Verification items for the finished model (mm, model axes). Give positions to 0.01 mm unless a question says otherwise; leave off trailing zeros. Loops run counter-clockwise (first coordinate to the right, second up) from the corner with the lowest first, then second, coordinate; pieces in that order, holes last. Notation, with made-up numbers: (73, 36.25) - (122, 36.25) arc R28 cw to (122, 69.25) - close; hole circle Ø9 at (-11.75, 73). An arc over 180 degrees is marked (long way). Answer in a Markdown table with one row per item.
```python
from build123d import *

# Parameters (mm, degrees)
SKETCH1_R           = 11.43
BOSS_EXTRUDE1_DEPTH = 2
SKETCH2_W           = 17.3
SKETCH2_H           = 1
SKETCH2_W_2         = 1
SKETCH2_H_2         = 17.3
CUT_EXTRUDE7_DEPTH  = 2
SKETCH3_R           = 9.65
BOSS_EXTRUDE2_DEPTH = 10
SKETCH4_R           = 8.65
CUT_EXTRUDE8_DEPTH  = 10


with BuildPart() as part:
    # Sketch1 → Boss-Extrude1 (new body)
    with BuildSketch(Plane(origin=(0, 0, 0), x_dir=(1, 0, 0), z_dir=(0, 1, 0))):
        with Locations(Location((0, 0, 0), (0, 0, 270))):
            Circle(SKETCH1_R)
    extrude(amount=BOSS_EXTRUDE1_DEPTH)

    # Sketch2 → Cut-Extrude7 (cut)
    with BuildSketch(Plane(origin=(0, 2, 0), x_dir=(1, 0, 0), z_dir=(0, 1, 0))):
        Polygon((-6.470027048, 5.762920267), (5.762920267, -6.470027048), (6.470027048, -5.762920267), (-5.762920267, 6.470027048), align=None)
        Rectangle(SKETCH2_W, SKETCH2_H)
        Rectangle(SKETCH2_W_2, SKETCH2_H_2)
        Polygon((5.762920267, 6.470027048), (-6.470027048, -5.762920267), (-5.762920267, -6.470027048), (6.470027048, 5.762920267), align=None)
    extrude(amount=-CUT_EXTRUDE7_DEPTH, mode=Mode.SUBTRACT)

    # Sketch3 → Boss-Extrude2 (add)
    with BuildSketch(Plane(origin=(0, 2, 0), x_dir=(1, 0, 0), z_dir=(0, 1, 0))):
        with Locations(Location((0, 0, 0), (0, 0, 270))):
            Circle(SKETCH3_R)
    extrude(amount=BOSS_EXTRUDE2_DEPTH)

    # Sketch4 → Cut-Extrude8 (cut)
    with BuildSketch(Plane(origin=(0, 12, 0), x_dir=(1, 0, 0), z_dir=(0, 1, 0))):
        with Locations(Location((0, 0, 0), (0, 0, 270))):
            Circle(SKETCH4_R)
    extrude(amount=-CUT_EXTRUDE8_DEPTH, mode=Mode.SUBTRACT)


solid = part.part
```
Q1. Draft check along Z on faces 1 (the face through (8, 12, -4)), 2 (the face through (3, 2, 6)), 3 (the face through (-3.168, 1.014, 3.875)). Enter one of: +Z half, -Z half, draft (parallel to the pull), parting line (faces both ways), or undercut.
Completed:
| item | result |
|---|---|
| face 1 | draft |
| face 2 | undercut |
| face 3 | undercut |
Q2. Sectioned sample at B-B (z = 5). Record the cut outline in (x, y), and give its area (3 significant figures).
Completed:
| item | result |
|---|---|
| outline | (-10.28, 0) - (-5.71, 0) - (-5.71, 2) - (-7.06, 2) - (-7.06, 12) - (-8.25, 12) - (-8.25, 2) - (-10.28, 2) - close; (-4.29, 0) - (-0.5, 0) - (-0.5, 2) - (-4.29, 2) - close; (0.5, 0) - (4.29, 0) - (4.29, 2) - (0.5, 2) - close; (5.71, 0) - (10.28, 0) - (10.28, 2) - (8.25, 2) - (8.25, 12) - (7.06, 12) - (7.06, 2) - (5.71, 2) - close |
| area | 57.4 mm^2 |
Q3. Sectioned sample at D-D (x = -8). Record the cut outline in (y, z).
Completed:
| item | result |
|---|---|
| outline | (0, -8.16) - (2, -8.16) - (2, -5.4) - (12, -5.4) - (12, -3.29) - (2, -3.29) - (2, -0.5) - (0, -0.5) - close; (0, 0.5) - (2, 0.5) - (2, 3.29) - (12, 3.29) - (12, 5.4) - (2, 5.4) - (2, 8.16) - (0, 8.16) - close |
Q4. Go/stop test with flat-tipped pins: P1, Ø2.5, axis at x = 3.5, z = 4, coming from the +Y side; P2, Ø1, axis at x = 4.5, y = 1.5, coming from the +Z side; P3, Ø1.5, axis at y = 10.5, z = 3, coming from the -X side. Record where each tip stops, or that it passes through.
Completed:
| item | result |
|---|---|
| P1 | y = 2 |
| P2 | z = 10.71 |
| P3 | x = -9.38 |
Q5. Thickness scan on line 1 (X direction, y = 6.5, z = 0); line 2 (Y direction, x = -8.25, z = -7). Record the ranges inside material, lowest first.
Completed:
| item | result |
|---|---|
| line 1 | -9.65 to -8.65, 8.65 to 9.65 |
| line 2 | 0 to 2 |
Q6. Sectioned sample at A-A (x = -4.25). Record the cut outline in (y, z), and give its area (3 significant figures).
Completed:
| item | result |
|---|---|
| outline | (0, -10.61) - (2, -10.61) - (2, -8.66) - (12, -8.66) - (12, -7.53) - (2, -7.53) - (2, -4.96) - (0, -4.96) - close; (0, -3.54) - (2, -3.54) - (2, -0.5) - (0, -0.5) - close; (0, 0.5) - (2, 0.5) - (2, 3.54) - (0, 3.54) - close; (0, 4.96) - (2, 4.96) - (2, 7.53) - (12, 7.53) - (12, 8.66) - (2, 8.66) - (2, 10.61) - (0, 10.61) - close |
| area | 57.4 mm^2 |
Q7. Sectioned sample at C-C (y = 9.75). Record the cut outline in (x, z), and give its area (3 significant figures).
Completed:
| item | result |
|---|---|
| outline | circle Ø19.3 at (0, 0); hole circle Ø17.3 at (0, 0) |
| area | 57.5 mm^2 |
